```python
from build123d import *


with BuildPart() as part:
    # Esquisse1 → Revolution1 (revolve)
    with BuildSketch(Plane.XY):
        Polygon((0, 0), (-20, 0), (-20, 3), (-23, 3), (-23, 4.5), (-19.5, 4.5), (-18.5, 3.5), (-17, 3.5), (-16, 4.5), (-15, 4.5), (-15, 2.25), (15, 2.25), (15, 4.5), (16, 4.5), (17, 3.5), (18.5, 3.5), (19.5, 4.5), (23, 4.5), (23, 3), (20, 3), (20, 0), align=None)
    revolve(axis=Axis((0, 0, 0), (-1, 0, 0)))


solid = part.part
```
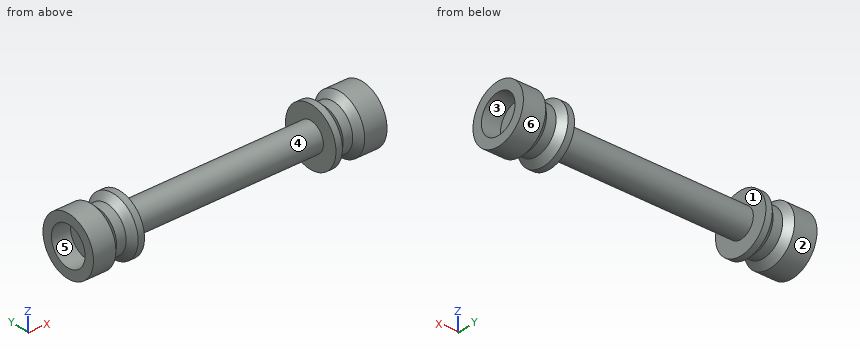
For this review, take the finished solid that the model builds, in its own axes (mm). Face numbers are marked on the shaded views. A direction names the side the tool comes from. Round coordinates to 2 decimals unless told otherwise and drop trailing zeros. Write each loop counter-clockwise with the first axis right and the second up, starting at its lowest first coordinate (ties: lowest second). Pieces come first, ordered by that corner, then holes. Notation, with made-up numbers: (11.25, 24) -> (59.25, 24) arc R22 ccw to (59.25, 62) -> close; hole circle Ø9 at (69.5, 36). An arc over 180 degrees is marked (long way). One line per question, with ' | ' between items. Start each with the question number.
(1) Add section A-A, the plane z = 4. Give the number of separate pieces and of enclosed holes in the cut face, plus the area to 3 significant figures.
(2) Insertion check: P1, Ø5, axis at y = -1, z = 1, coming from the -X side; P2, Ø1.5, axis at x = 7, y = 1, coming from the +Z side; P3, Ø5, axis at x = 17, y = -3, coming from the +Z side; P4, Ø4, axis at x = 5.5, z = -2.5, coming from the -Y side. Each pin has a flat end and moves straight along its axis. Give the tip position at first contact, or say it passes through.
(3) Tool access review of the marked faces 4, 5 and 6: name each direction out of +Z, -Z, +X, -X, +Y, -Y from which nothing blocks a thin tool from reaching the whole face with its end or side.
(4) Add section B-B, the plane x = 12.5. Write out the cut boundary in (y, z), plus the area to 3 significant figures.
(5) Mouldability with a two-part tool opening along Y and no side actions: class the marked faces 1, 2 and 3 as released by +Y, released by -Y, zero draft, split by the parting line, or undercut.
(6) For line 1 along Z through (x, y) = (-21.4, 0); line 2 along X through (y, z) = (-2.5, -1.75), list the stretches that pass through material, from the lowest coordinate up. Write a range as from..to.
Answer list:
1) separate pieces: 4 | enclosed holes: 0 | area: 42.5 mm²
2) P1: x = -23 | P2: z = 2.24 | P3: z = 4.44 | P4: y = -2.19
3) face 4: none | face 5: -X | face 6: +X, -X
4) outline: circle Ø4.5 at (0, 0) | area: 15.9 mm²
5) face 1: zero draft | face 2: split by the parting line | face 3: undercut
6) line 1: -4.5..-3, 3..4.5 | line 2: -23..-15, 15..23
